```python
from build123d import *

# Parameters (mm, degrees)
SKETCH1_W                          = 7.25
SKETCH1_H                          = 18
BOSS_EXTRUDE1_DEPTH                = 23
CUT_EXTRUDE1_DEPTH                 = 1
CUT_EXTRUDE1_DEPTH_BACK            = 8.25
M2_5X0_45_TAPPED_HOLE1_D           = 2.05
M2_5X0_45_TAPPED_HOLE1_DEPTH       = 6.35
M2_5X0_45_TAPPED_HOLE1_TIP         = 0.615882135
M2_5X0_45_TAPPED_HOLE2_D           = 2.05
M2_5X0_45_TAPPED_HOLE2_DEPTH       = 6.35
M2_5X0_45_TAPPED_HOLE2_TIP         = 0.615882135
M2_5X0_45_TAPPED_HOLE3_D           = 2.05
M2_5X0_45_TAPPED_HOLE3_DEPTH       = 6.35
M2_5X0_45_TAPPED_HOLE3_CBORE_D     = 2.5
M2_5X0_45_TAPPED_HOLE3_CBORE_DEPTH = 5
M2_5X0_45_TAPPED_HOLE3_TIP         = 0.615882135
FILLET1_R                          = 3


with BuildPart() as part:
    # Sketch1 → Boss-Extrude1 (new body)
    with BuildSketch(Plane(origin=(0, 0, 0), x_dir=(1, 0, 0), z_dir=(0, 1, 0))):
        Rectangle(SKETCH1_W, SKETCH1_H)
    extrude(amount=BOSS_EXTRUDE1_DEPTH)

    # Sketch2 → Cut-Extrude1 (cut, two sides)
    with BuildSketch(Plane.ZY.offset(3.625)) as cut_extrude1_sk:
        Polygon((-77.412327466, 23), (-9, 23), (-2, 23), (2, 17.5), (9, 17.5), (77.412327466, 17.5), (82.269830407, 154.238403027), (-72.554824525, 159.738403027), align=None)
    extrude(amount=CUT_EXTRUDE1_DEPTH, mode=Mode.SUBTRACT)
    extrude(cut_extrude1_sk.sketch, amount=-CUT_EXTRUDE1_DEPTH_BACK, mode=Mode.SUBTRACT)

    # M2.5x0.45 Tapped Hole1
    with Locations(Plane(origin=(0, 0, 0), x_dir=(-1, 0, 0), z_dir=(0, -1, 0))):
        with Locations((0, 0)):
            Hole(M2_5X0_45_TAPPED_HOLE1_D / 2, depth=M2_5X0_45_TAPPED_HOLE1_DEPTH)
            with Locations((0, 0, -(M2_5X0_45_TAPPED_HOLE1_DEPTH + M2_5X0_45_TAPPED_HOLE1_TIP / 2))):  # 118° drill point
                Cone(0, M2_5X0_45_TAPPED_HOLE1_D / 2, M2_5X0_45_TAPPED_HOLE1_TIP, mode=Mode.SUBTRACT)

    # M2.5x0.45 Tapped Hole2
    with Locations(Plane(origin=(0, 23, 0), x_dir=(1, 0, 0), z_dir=(0, 1, 0))):
        with Locations((0, 5.5)):
            Hole(M2_5X0_45_TAPPED_HOLE2_D / 2, depth=M2_5X0_45_TAPPED_HOLE2_DEPTH)
            with Locations((0, 0, -(M2_5X0_45_TAPPED_HOLE2_DEPTH + M2_5X0_45_TAPPED_HOLE2_TIP / 2))):  # 118° drill point
                Cone(0, M2_5X0_45_TAPPED_HOLE2_D / 2, M2_5X0_45_TAPPED_HOLE2_TIP, mode=Mode.SUBTRACT)

    # M2.5x0.45 Tapped Hole3
    with Locations(Plane(origin=(0, 17.5, 0), x_dir=(1, 0, 0), z_dir=(0, 1, 0))):
        with Locations((0, -5.5)):
            CounterBoreHole(M2_5X0_45_TAPPED_HOLE3_D / 2, M2_5X0_45_TAPPED_HOLE3_CBORE_D / 2, M2_5X0_45_TAPPED_HOLE3_CBORE_DEPTH, depth=M2_5X0_45_TAPPED_HOLE3_DEPTH)
            with Locations((0, 0, -(M2_5X0_45_TAPPED_HOLE3_DEPTH + M2_5X0_45_TAPPED_HOLE3_TIP / 2))):  # 118° drill point
                Cone(0, M2_5X0_45_TAPPED_HOLE3_D / 2, M2_5X0_45_TAPPED_HOLE3_TIP, mode=Mode.SUBTRACT)

    # Fillet1
    fillet1_edges = [part.edges().sort_by_distance(p)[0] for p in [
        (3.625, 8.75, 9),
        (-3.625, 8.75, 9),
        (-3.625, 11.5, -9),
        (3.625, 11.5, -9),
    ]]
    fillet(fillet1_edges, radius=FILLET1_R)


solid = part.part
```
Here's how the part is built. I have some questions about the finished solid (model axes, mm). A direction names the side the tool comes from. Give positions to 0.01 mm unless a question says otherwise; leave off trailing zeros. Loops run counter-clockwise (first coordinate to the right, second up) from the corner with the lowest first, then second, coordinate; pieces in that order, holes last. Notation, with made-up numbers: M 44,16 L 52,16 A35 cw 52,51 Z; hole C 63.5,23 d4. An arc over 180 degrees is marked long. Return JSON: item names as keys, results as strings.
Item 1: Imagine slicing it at C-C on y = 21.25. List the corners of the cut face in (x, z) for me (3 decimals).
A:
{"outline": "M -3.625,-6 A3 ccw -0.625,-9 L 0.625,-9 A3 ccw 3.625,-6 L 3.625,-0.727 L -3.625,-0.727 Z; hole C 0,-5.5 d2.05"}
Item 2: Imagine slicing it at A-A on y = 11.5. List the corners of the cut face in (x, z) for me (3 decimals), then the cut area to 3 significant figures.
A:
{"outline": "M -3.625,-6 A3 ccw -0.625,-9 L 0.625,-9 A3 ccw 3.625,-6 L 3.625,6 A3 ccw 0.625,9 L -0.625,9 A3 ccw -3.625,6 Z; hole C 0,5.5 d2.05", "area": "119 mm^2"}
Item 3: Imagine slicing it at D-D on x = -2.5. List the corners of the cut face in (y, z) for me, then the cut area to 3 significant figures.
A:
{"outline": "M 0,-8.34 L 23,-8.34 L 23,-2 L 17.5,2 L 17.5,8.34 L 0,8.34 Z", "area": "338 mm^2"}
Item 4: On a 3-axis mill with a long thin cutter (end or side, diameter ignored), from which of +Z, -Z, +X, -X, +Y, -Y can I reach the whole of each face in a straight line? I mean faces 1 (the cylindrical face through (-0.27, 15.04, 6.72)), 2 (the flat face through (0, 17.5, 4)), 3 (the cylindrical face through (-0.133, 3.219, -1.016)). Say none if no direction works.
A:
{"face 1": "+Y", "face 2": "+Z, +X, -X, +Y", "face 3": "-Y"}
Item 5: I'm going to push flat-ended pins straight in: pin 1 Ø0.8 at (x, z) = (-0.5, 5) entering from +Y; pin 2 Ø3 at (x, y) = (-1, 20) entering from +Z; pin 3 Ø1.2 at (x, z) = (0, 0) entering from +Y (3 decimals). Where does each tip first touch, or does it pass through?
A:
{"pin 1": "stops at y = 12.5", "pin 2": "stops at z = 1.27", "pin 3": "stops at y = 21.075"}
Item 6: Please list where these lines run through material, in increasing order: line 1 (X direction, y = 14, z = 5.5) (3 decimals); line 2 (Z direction, x = 0, y = 2.75) (3 decimals); line 3 (Z direction, x = 0, y = 15.6).
A:
{"line 1": "x = -3.625 to -1.25, 1.25 to 3.625", "line 2": "z = -9 to -1.025, 1.025 to 9", "line 3": "z = -9 to 4.25, 6.75 to 9"}
Item 7: Thinking about a two-plate mould opening in Z: for faces 4 (the flat face through (-3.625, 11, 0)), 5 (the flat face through (0, 9, 9)), 6 (the cylindrical face through (0.22, 19.78, -4.5)), which applies, released by +Z, released by -Z, zero draft, split by the parting line, or undercut?
A:
{"face 4": "zero draft", "face 5": "released by +Z", "face 6": "undercut"}
Item 8: Imagine slicing it at B-B on x = 2. List the corners of the cut face in (y, z) for me.
A:
{"outline": "M 0,-8.67 L 23,-8.67 L 23,-2 L 17.5,2 L 17.5,8.67 L 0,8.67 Z"}
